Geometry check sheet. Reference: the model listing, model coordinates, mm. A direction names the side the tool comes from. Round coordinates to 2 decimals unless told otherwise and drop trailing zeros. Order: outer loops, then holes, each group sorted by start corner. A loop starts at its lowest first (then second) coordinate and runs counter-clockwise, first axis right, second up. Notation, with made-up numbers: (-19.75, 42.5) - (12.25, 42.5) arc R4 ccw to (12.25, 49.5) - close; hole circle Ø1 at (12.25, -36.5). An arc over 180 degrees is marked (long way). Use a Markdown table: item, result. Add a question column.
(1) Mould release check, pull along X, two halves, no side actions. Record for faces 4 (the face through (9.43, 0.31, 83.1)), 5 (the face through (6, 0, 12)), 6 (the face through (-11.417, 0.308, 11.717)): released by +X, released by -X, zero draft, split by the parting line, or undercut.
(2) Section check D-D on x = -9. Record the boundary of the cut face in (y, z), then the cut area to 3 significant figures.
(3) Section check A-A on x = 3.5. Record the boundary of the cut face in (y, z).
(4) Section check C-C on z = 48. Record the boundary of the cut face in (x, y), then the cut area to 3 significant figures.
(5) Access from +Z, -Z, +X, -X, +Y, -Y to the whole of each face (thin tool, end or side, straight path). Record for faces 1 (the face through (10, 0, 88)), 2 (the face through (-10, 0, 52)), 3 (the face through (0, 0, 11)).
(6) Thickness scan on line 1 along Z through (x, y) = (-3.5, -19); line 2 along X through (y, z) = (4.5, 17.5); line 3 along X through (y, z) = (-12.5, 7). Record the ranges inside material, lowest first. Write a range as [from, to].
(7) Gauge pin test, flat ends, axial feed: P1, Ø8, axis at y = 4.5, z = 66, coming from the -X side; P2, Ø5.5, axis at y = 5, z = 87.5, coming from the +X side; P3, Ø6, axis at y = 13, z = 32.5, coming from the +X side; P4, Ø12, axis at x = 1.5, z = 36, coming from the -Y side. Record the tip position at first contact, or that the pin passes through.
```python
from build123d import *

# Parameters (mm, degrees)
F0_W         = 39
F0_H         = 44
F1_DEPTH     = 7
F3_DEPTH     = 44
F4_W         = 20
F4_H         = 44
F5_DEPTH     = 5
F6_W         = 20
F6_H         = 44
F7_DEPTH     = 79.5
F8_W         = 12
F8_H         = 76.5
F9_DEPTH     = 44
F10_W        = 4
F10_H        = 66.5
F11_DEPTH    = 44
F12_R        = 1.99999
F13_T1_DEPTH = 44
F14_R        = 5


# Not quite as in the source:
# - a fillet or chamfer that OpenCascade refuses, or shapes differently, is made with other operations: its cross-section is extruded or revolved along the edge and cut away or added
# - a fillet or chamfer is up to 0.001 mm smaller than in the source, because OpenCascade refuses the exact size


with BuildPart() as f1:
    # F0 (on Top) → F1 (new body)
    with BuildSketch(Plane.XY):
        Rectangle(F0_W, F0_H)
    extrude(amount=F1_DEPTH)

    # F2 (on face) → F3 (cut)
    with BuildSketch(Plane.XZ.offset(22)):
        Polygon((-19.5, 7), (-19.5, 0), (-15.5, 7), align=None)
        Polygon((16.5, 7), (19.5, 0), (19.5, 7), align=None)
    extrude(amount=-F3_DEPTH, mode=Mode.SUBTRACT)

    # F4 (on face) → F5 (join)
    with BuildSketch(Plane.XY.offset(7)):
        Rectangle(F4_W, F4_H)
    extrude(amount=F5_DEPTH)

    # F6 (on face) → F7 (join)
    with BuildSketch(Plane.XY.offset(12)):
        Rectangle(F6_W, F6_H)
    extrude(amount=F7_DEPTH)

    # F8 (on face) → F9 (cut)
    with BuildSketch(Plane.XZ.offset(22)):
        with Locations((0, 49.25)):
            Rectangle(F8_W, F8_H)
    extrude(amount=-F9_DEPTH, mode=Mode.SUBTRACT)

    # F10 (on face) → F11 (cut)
    with BuildSketch(Plane.XZ.offset(22)):
        with Locations((8, 49.25)):
            Rectangle(F10_W, F10_H)
    extrude(amount=-F11_DEPTH, mode=Mode.SUBTRACT)

    # F12 (radius 2 in the source; OpenCascade refuses exactly that, so slightly less here)
    f12_edges = [f1.edges().sort_by_distance(p)[0] for p in [
        (10, 0, 82.5),
        (6, 0, 16),
        (10, 0, 16),
        (6, 0, 82.5),
    ]]
    fillet(f12_edges, radius=F12_R)

    # F13: fillet of radius 13 on 2 edges, made by hand

    # F13_s2 → F13_t1 (join)
    with BuildSketch(Plane.XZ.offset(-22)):
        with BuildLine():
            ThreePointArc((16.5, 7), (12.4319250008, 10.1446687277), (9.9012785359, 14.6206048393))
            Line((9.9012785359, 14.6206048393), (8.6654478084, 14.2172161768))
            ThreePointArc((8.6654478084, 14.2172161768), (8.7, 14.00001), (8.7, 7))
            Line((8.7, 7), (10, 5.7))
            ThreePointArc((10, 5.7), (13.25, 5.7), (15.9240414189, 5.8345508536))
            Line((15.9240414189, 5.8345508536), (16.5, 7))
        make_face()
        with BuildLine():
            ThreePointArc((-10, 17.6183802908), (-11.4566036194, 11.6392499192), (-15.5, 7))
            Line((-15.5, 7), (-15.35, 6.7876323942))
            ThreePointArc((-15.35, 6.7876323942), (-12.75, 6.74), (-10, 6.74))
            Line((-10, 6.74), (-9.74, 7))
            Line((-9.74, 7), (-9.74, 17.6183802908))
            Line((-9.74, 17.6183802908), (-10, 17.6183802908))
        make_face()
    extrude(amount=F13_T1_DEPTH)

    # F14
    f14_edges = [f1.edges().sort_by_distance(p)[0] for p in [
        (-10, 0, 91.5),
    ]]
    fillet(f14_edges, radius=F14_R)


solid = f1.part
```
Check sheet entries:
| question | item | result |
|---|---|---|
| 1 | face 4 | released by +X |
| 1 | face 5 | undercut |
| 1 | face 6 | released by -X |
| 2 | outline | (-22, 0) - (22, 0) - (22, 89.5) - (-22, 89.5) - close |
| 2 | area | 3,940 mm2 |
| 3 | outline | (-22, 0) - (22, 0) - (22, 11) - (-22, 11) - close; (-22, 87.5) - (22, 87.5) - (22, 91.5) - (-22, 91.5) - close |
| 4 | outline | (-10, -22) - (-6, -22) - (-6, 22) - (-10, 22) - close |
| 4 | area | 176 mm2 |
| 5 | face 1 | +Z, +X, +Y, -Y |
| 5 | face 2 | +Z, -X, +Y, -Y |
| 5 | face 3 | +Y, -Y |
| 6 | line 1 | z = [0, 11], [87.5, 91.5] |
| 6 | line 2 | x = [-10, -6] |
| 6 | line 3 | x = [-15.5, 16.5] |
| 7 | P1 | stops at x = -10 |
| 7 | P2 | stops at x = 10 |
| 7 | P3 | stops at x = -6 |
| 7 | P4 | passes through |
